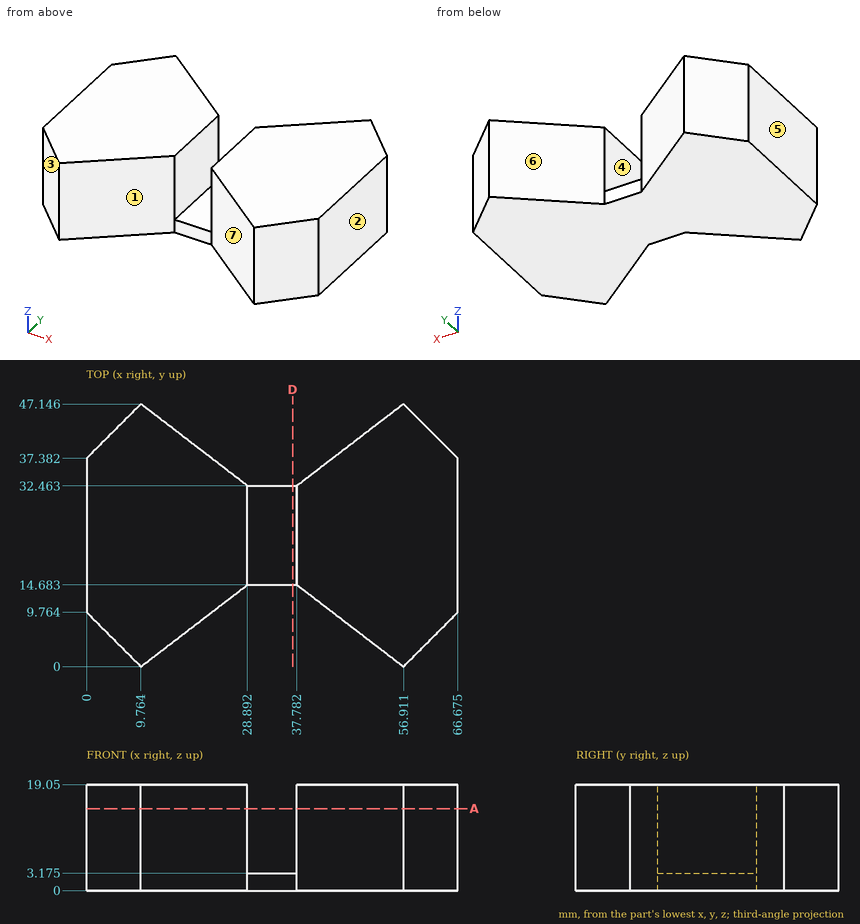
Geometry check sheet. Reference: drawing and pictorial views, mm from the part's lowest x, y, z. A direction names the side the tool comes from. Coordinates: 2 decimals unless noted, no trailing zeros. Order: outer loops, then holes, each group sorted by start corner. A loop starts at its lowest first (then second) coordinate and runs counter-clockwise, first axis right, second up. Notation, with made-up numbers: (68, 49) - (82, 49) arc R8 cw to (82, 59) - close; hole circle Ø6 at (-30.75, 36.25). An arc over 180 degrees is marked (long way). One line per item, written item: value.
(1) Depth check by flat-ended pin: pin 1 Ø3.5 at (x, z) = (34.5, 1.5) entering from +Y; pin 2 Ø4 at (x, z) = (55.5, 9.5) entering from -Y; pin 3 Ø3.5 at (x, z) = (31.5, 1) entering from -Y. Enter the tip coordinate at first touch or a pass-through.
Data:
pin 1: stops at y = 32.46
pin 2: stops at y = 0
pin 3: stops at y = 14.68
(2) Sectioned sample at D-D (x = 37). Enter the section's corners in (y, z) (1 decimal).
Data:
outline: (14.7, 0) - (32.5, 0) - (32.5, 3.2) - (14.7, 3.2) - close
(3) Thickness scan on probe 1 along X at (y, z) = (22.5, 14.25) (1 decimal); probe 2 along X at (y, z) = (36, 15.25) (1 decimal); probe 3 along Z at (x, y) = (35, 19.5) (1 decimal). Record the ranges inside material, lowest first. Write a range as from..to.
Data:
probe 1: x = 0..28.9, 37.8..66.7
probe 2: x = 0..24.3, 42.4..66.7
probe 3: z = 0..3.2
(4) Access from +Z, -Z, +X, -X, +Y, -Y to the whole of each face (thin tool, end or side, straight path). Record for the marked faces 4, 5, 6 and 7.
Data:
face 4: +Z, +Y, -Y
face 5: +Z, -Z, -X, +Y, -Y
face 6: +Z, -Z, +Y
face 7: +Z, -Z, -Y
(5) Sectioned sample at A-A (z = 14.75). Enter the section's corners in (x, y) (1 decimal).
Data:
outline: (0, 9.8) - (9.8, 0) - (28.9, 14.7) - (28.9, 32.5) - (9.8, 47.1) - (0, 37.4) - close; (37.8, 14.7) - (56.9, 0) - (66.7, 9.8) - (66.7, 37.4) - (56.9, 47.1) - (37.8, 32.5) - close
(6) Release check for a two-part mould opening along X. For the marked faces 1, 2 and 3 record: +X half, -X half, draft (parallel to the pull), parting line (faces both ways), or undercut.
Data:
face 1: undercut
face 2: +X half
face 3: -X half
